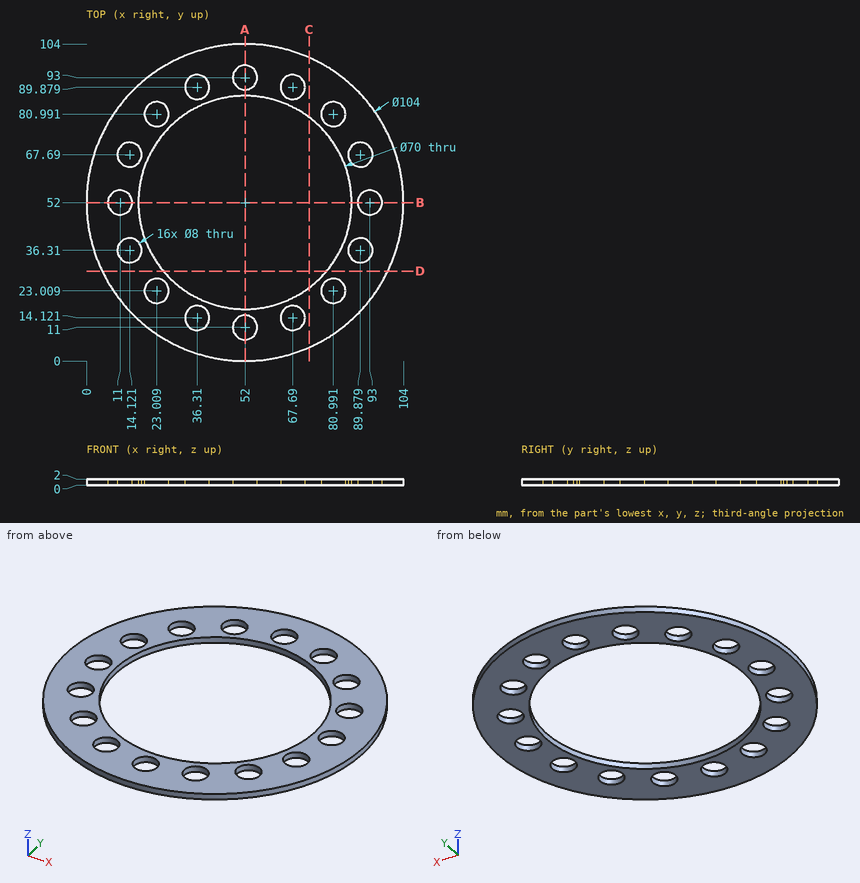
Design review of the part shown in the three views and the two pictorial views. Dimensions are in mm from the part's minimum x, y and z. Coordinates: 2 decimals unless noted, no trailing zeros. Order: outer loops, then holes, each group sorted by start corner. A loop starts at its lowest first (then second) coordinate and runs counter-clockwise, first axis right, second up.
1) Take a section at C-C, the plane x = 73. Give the boundary of the cut face in (y, z).
2) Clearance check with a flat-ended pin moving along its axis: pin 1 (5 mm diameter, centred on x = 23.01, y = 80.99, fed in from +Z). State where the tip first meets the part, or that it passes through.
3) Take a section at A-A, the plane x = 52. Give the boundary of the cut face in (y, z).
4) Take a section at D-D, the plane y = 29.5. Give the boundary of the cut face in (x, z).
5) Wall thickness on line 1 along X through (y, z) = (51, 1.75) (1 decimal); line 2 along Y through (x, z) = (10.5, 1.45) (1 decimal); line 3 along Y through (x, z) = (70, 0.55) (1 decimal): over which ranges is each line inside the solid? List them lowest first.
Returned:
1. outline: (4.43, 0) - (24, 0) - (24, 2) - (4.43, 2) - close; (80, 0) - (99.57, 0) - (99.57, 2) - (80, 2) - close
2. pin 1: passes through
3. outline: (0, 0) - (7, 0) - (7, 2) - (0, 2) - close; (15, 0) - (17, 0) - (17, 2) - (15, 2) - close; (87, 0) - (89, 0) - (89, 2) - (87, 2) - close; (97, 0) - (104, 0) - (104, 2) - (97, 2) - close
4. outline: (5.12, 0) - (25.19, 0) - (25.19, 2) - (5.12, 2) - close; (78.81, 0) - (98.88, 0) - (98.88, 2) - (78.81, 2) - close
5. line 1: x = 0 to 7.1, 14.9 to 17, 87 to 89.1, 96.9 to 104
5. line 2: y = 20.7 to 34.6, 38 to 48, 56 to 66, 69.4 to 83.3
5. line 3: y = 3.2 to 10.9, 17.4 to 22, 82 to 86.6, 93.1 to 100.8
